from build123d import *

# Parameters (mm, degrees)
SKETCH1_W           = 65
SKETCH1_H           = 82.5
BOSS_EXTRUDE1_DEPTH = 10
SKETCH2_W           = 63
SKETCH2_H           = 80.5
CUT_EXTRUDE1_DEPTH  = 9
SKETCH4_R           = 2.5
BOSS_EXTRUDE2_DEPTH = 2.5
SKETCH5_W           = 7.5
SKETCH5_H           = 4
CUT_EXTRUDE2_DEPTH  = 1


with BuildPart() as part:
    # Sketch1 → Boss-Extrude1 (new body)
    with BuildSketch(Plane(origin=(0, 0, 0), x_dir=(1, 0, 0), z_dir=(0, 1, 0))):
        Rectangle(SKETCH1_W, SKETCH1_H)
    extrude(amount=BOSS_EXTRUDE1_DEPTH)

    # Sketch2 → Cut-Extrude1 (cut)
    with BuildSketch(Plane(origin=(0, 10, 0), x_dir=(1, 0, 0), z_dir=(0, 1, 0))):
        Rectangle(SKETCH2_W, SKETCH2_H)
    extrude(amount=-CUT_EXTRUDE1_DEPTH, mode=Mode.SUBTRACT)

    # Sketch4 → Boss-Extrude2 (add)
    with BuildSketch(Plane(origin=(0, 1, 0), x_dir=(1, 0, 0), z_dir=(0, 1, 0))):
        with Locations((-28, 36.75)):
            Circle(SKETCH4_R)
        with Locations((28, 36.75)):
            Circle(SKETCH4_R)
        with Locations((-28, -36.75)):
            Circle(SKETCH4_R)
        with Locations((28, -36.75)):
            Circle(SKETCH4_R)
        Circle(SKETCH4_R)
    extrude(amount=BOSS_EXTRUDE2_DEPTH)

    # Sketch5 → Cut-Extrude2 (cut)
    with BuildSketch(Plane.ZY.offset(32.5)):
        with Locations((3, 6)):
            Rectangle(SKETCH5_W, SKETCH5_H)
    extrude(amount=-CUT_EXTRUDE2_DEPTH, mode=Mode.SUBTRACT)


solid = part.part
Geometry: final body of the model. Coordinates: model frame, mm. A direction names the side the tool comes from. Give positions to 0.01 mm unless a question says otherwise; leave off trailing zeros. Order: outer loops, then holes, each group sorted by start corner. A loop starts at its lowest first (then second) coordinate and runs counter-clockwise, first axis right, second up. Notation, with made-up numbers: (68, -32.75) -> (108, -32.75) arc R25 ccw to (108, -8.75) -> close; hole circle Ø10 at (87, -21). An arc over 180 degrees is marked (long way). Put each result on its own line as item: value.
Q1. Draft query along Z for faces 3 (the face through (0, 5, -41.25)), 4 (the face through (0, 0, -1)), 5 (the face through (0, 6, -40.25)). Return one class per face: released by +Z, released by -Z, zero draft, split by the parting line, or undercut.
Here are the results:
face 3: released by -Z
face 4: zero draft
face 5: undercut
Q2. Pin query (flat end, axial travel): pin 1 (1.5 mm diameter, centred on x = 29, z = 37, fed in from +Y); pin 2 (1 mm diameter, centred on x = -7.5, z = -8.5, fed in from +Y). Return the tip coordinate at first contact, or that it passes through.
Here are the results:
pin 1: stops at y = 3.5
pin 2: stops at y = 1
Q3. Section D-D, the plane x = -28. Return loops of the section in (y, z).
Here are the results:
outline: (0, -41.25) -> (10, -41.25) -> (10, -40.25) -> (1, -40.25) -> (1, -39.25) -> (3.5, -39.25) -> (3.5, -34.25) -> (1, -34.25) -> (1, 34.25) -> (3.5, 34.25) -> (3.5, 39.25) -> (1, 39.25) -> (1, 40.25) -> (10, 40.25) -> (10, 41.25) -> (0, 41.25) -> close
Q4. Section B-B, the plane y = 7. Return loops of the section in (x, z).
Here are the results:
outline: (-32.5, -41.25) -> (32.5, -41.25) -> (32.5, 41.25) -> (-32.5, 41.25) -> (-32.5, 6.75) -> (-31.5, 6.75) -> (-31.5, 40.25) -> (31.5, 40.25) -> (31.5, -40.25) -> (-31.5, -40.25) -> (-31.5, -0.75) -> (-32.5, -0.75) -> close
Q5. Material intervals for L1, parallel to Z at x = -9, y = 8.5; L2, parallel to X at y = 7.75, z = -2; L3, parallel to Z at x = 28.5, y = 3.25, sorted ascending.
Here are the results:
L1: z = -41.25 to -40.25, 40.25 to 41.25
L2: x = -32.5 to -31.5, 31.5 to 32.5
L3: z = -41.25 to -40.25, -39.2 to -34.3, 34.3 to 39.2, 40.25 to 41.25
Q6. Section C-C, the plane z = 29.5. Return loops of the section in (x, y), then the cut area to 3 significant figures.
Here are the results:
outline: (-32.5, 0) -> (32.5, 0) -> (32.5, 10) -> (31.5, 10) -> (31.5, 1) -> (-31.5, 1) -> (-31.5, 10) -> (-32.5, 10) -> close
area: 83.0 mm^2
Q7. Section A-A, the plane x = 0. Return loops of the section in (y, z).
Here are the results:
outline: (0, -41.25) -> (10, -41.25) -> (10, -40.25) -> (1, -40.25) -> (1, -2.5) -> (3.5, -2.5) -> (3.5, 2.5) -> (1, 2.5) -> (1, 40.25) -> (10, 40.25) -> (10, 41.25) -> (0, 41.25) -> close
Q8. Reachability of faces 1 (the face through (-32.5, 3.8, 0.6)), 2 (the face through (31.5, 6, 1)) from +Z, -Z, +X, -X, +Y, -Y: full face, straight path, thin tool, end or side. Return the list, or none.
Here are the results:
face 1: +Z, -Z, -X, +Y, -Y
face 2: +Y
